Read the model definition and answer for the solid it produces. Units are mm, in the model's axes. A direction names the side the tool comes from. Give positions to 0.01 mm unless a question says otherwise; leave off trailing zeros. Loops run counter-clockwise (first coordinate to the right, second up) from the corner with the lowest first, then second, coordinate; pieces in that order, holes last. Notation, with made-up numbers: (-27, 4.5) - (6, 4.5) arc R31 cw to (6, 43.5) - close; hole circle Ø9 at (57, -15). An arc over 180 degrees is marked (long way). Write item = value, one per line. Start each with the question number.
from build123d import *

# Parameters (mm, degrees)
EXTRUDE_1_DEPTH = 6
FILLET_1_R      = 3
CHAMFER_1_SIZE  = 3


with BuildPart() as part:
    # 草图1 → 凸台-拉伸1 (new body)
    with BuildSketch(Plane.XY):
        Polygon((-50, 0), (50, 0), (50, 10), (9, 10), (9, 19), (-9, 19), (-9, 10), (-50, 10), align=None)
    extrude(amount=EXTRUDE_1_DEPTH)

    # 圆角1
    fillet_1_edges = [part.edges().sort_by_distance(p)[0] for p in [
        (50, 10, 3),
        (50, 0, 3),
        (-50, 0, 3),
        (-50, 10, 3),
    ]]
    fillet(fillet_1_edges, radius=FILLET_1_R)

    # 倒角1
    chamfer_1_edges = [part.edges().sort_by_distance(p)[0] for p in [
        (0, 19, 6),
        (0, 19, 0),
    ]]
    chamfer(chamfer_1_edges, length=CHAMFER_1_SIZE - 0.0001)  # a hair under: the kernel refuses the full size


solid = part.part
1. A cutting plane is placed at D-D on x = -21. Give the vertices of the cut face in (y, z).
2. Given P1, Ø3, axis at y = 14.5, z = 2.5, coming from the +X side; P2, Ø1.8, axis at x = 29.5, z = 2, coming from the +Y side, each flat-ended and moving along its own axis, determine where each tip first touches the part or whether it passes through.
3. A tool of negligible diameter and unlimited length cuts with its end or side. For faces 1 (the flat face through (0, 18, 2)), 2 (the flat face through (-9, 14, 3)), 3 (the flat face through (9, 13, 3)), from which of +Z, -Z, +X, -X, +Y, -Y can it reach the whole face along a straight path? Write none if from no direction.
4. A cutting plane is placed at B-B on z = 1.25. Give the vertices of the cut face in (x, y), and give its area (3 significant figures).
5. Consider line 1 along Y through (x, z) = (-39, 2); line 2 along X through (y, z) = (15.25, 1.5); line 3 along Y through (x, z) = (-6, 3.75). Determine where each line is inside the solid, lowest interval first. Write a range as [from, to].
6. A cutting plane is placed at C-C on y = 9. Give the vertices of the cut face in (x, z), and give its area (3 significant figures).
Reply:
q1.outline = (0, 0) - (10, 0) - (10, 6) - (0, 6) - close
q2.P1 = 9
q2.P2 = 10
q3.face_1 = -Z, +X, -X, +Y
q3.face_2 = +Z, -Z, -X, +Y
q3.face_3 = +Z, -Z, +X, +Y
q4.outline = (-50, 3) arc R3 ccw to (-47, 0) - (47, 0) arc R3 ccw to (50, 3) - (50, 7) arc R3 ccw to (47, 10) - (9, 10) - (9, 17.25) - (-9, 17.25) - (-9, 10) - (-47, 10) arc R3 ccw to (-50, 7) - close
q4.area = 1,120 mm^2
q5.line_1 = [0, 10]
q5.line_2 = [-9, 9]
q5.line_3 = [0, 18.25]
q6.outline = (-49.24, 0) - (49.24, 0) - (49.24, 6) - (-49.24, 6) - close
q6.area = 591 mm^2
